The listing builds one solid part. Answer for the finished solid, in the listing's coordinates (mm). A direction names the side the tool comes from. Round coordinates to 2 decimals unless told otherwise and drop trailing zeros. Loops run counter-clockwise (first coordinate to the right, second up) from the corner with the lowest first, then second, coordinate; pieces in that order, holes last. Notation, with made-up numbers: (79, 32) -> (97, 32) arc R31 cw to (97, 56) -> close; hole circle Ø2 at (10, 24). An arc over 180 degrees is marked (long way). Write each question's results on one line, items separated by ' | '. Start each with the question number.
from build123d import *

# Parameters (mm, degrees)
F1_DEPTH = 40
F3_DEPTH = 260


with BuildPart() as f1:
    # F0 (on Top) → F1 (new body)
    with BuildSketch(Plane.XY):
        with BuildLine():
            Line((184.88144, 231.240067), (-175.11856, 231.240067))
            ThreePointArc((-175.11856, 231.240067), (-189.260696, 225.382203), (-195.11856, 211.240067))
            Line((-195.11856, 211.240067), (-195.11856, -148.759933))
            ThreePointArc((-195.11856, -148.759933), (-189.260696, -162.902068), (-175.11856, -168.759933))
            Line((-175.11856, -168.759933), (184.88144, -168.759933))
            ThreePointArc((184.88144, -168.759933), (199.023575, -162.902068), (204.88144, -148.759933))
            Line((204.88144, -148.759933), (204.88144, 211.240067))
            ThreePointArc((204.88144, 211.240067), (199.023575, 225.382203), (184.88144, 231.240067))
        make_face()
    extrude(amount=F1_DEPTH)

    # F2 (on face) → F3 (join)
    with BuildSketch(Plane(origin=(0, 0, 0), x_dir=(1, 0, 0), z_dir=(0, 0, -1))):
        with BuildLine():
            ThreePointArc((-135.11856, -191.240067), (-120.976425, -185.382203), (-115.11856, -171.240067))
            ThreePointArc((-115.11856, -171.240067), (-120.976425, -157.097932), (-135.11856, -151.240067))
            ThreePointArc((-135.11856, -151.240067), (-149.260696, -157.097932), (-155.11856, -171.240067))
            ThreePointArc((-155.11856, -171.240067), (-149.260696, -185.382203), (-135.11856, -191.240067))
        make_face()
        with BuildLine():
            ThreePointArc((-135.11856, 88.759933), (-120.976425, 94.617797), (-115.11856, 108.759933))
            ThreePointArc((-115.11856, 108.759933), (-120.976425, 122.902068), (-135.11856, 128.759933))
            ThreePointArc((-135.11856, 128.759933), (-149.260696, 122.902068), (-155.11856, 108.759933))
            ThreePointArc((-155.11856, 108.759933), (-149.260696, 94.617797), (-135.11856, 88.759933))
        make_face()
        with BuildLine():
            ThreePointArc((144.88144, 128.759933), (130.739304, 122.902068), (124.88144, 108.759933))
            ThreePointArc((124.88144, 108.759933), (130.739304, 94.617797), (144.88144, 88.759933))
            ThreePointArc((144.88144, 88.759933), (159.023575, 94.617797), (164.88144, 108.759933))
            ThreePointArc((164.88144, 108.759933), (159.023575, 122.902068), (144.88144, 128.759933))
        make_face()
        with BuildLine():
            ThreePointArc((164.88144, -171.240067), (159.023575, -157.097932), (144.88144, -151.240067))
            ThreePointArc((144.88144, -151.240067), (130.739304, -157.097932), (124.88144, -171.240067))
            ThreePointArc((124.88144, -171.240067), (130.739304, -185.382203), (144.88144, -191.240067))
            ThreePointArc((144.88144, -191.240067), (159.023575, -185.382203), (164.88144, -171.240067))
        make_face()
    extrude(amount=F3_DEPTH)


solid = f1.part
Item 1: The part is cut by section D-D, the plane x = 40.5. Give the vertices of the cut face in (y, z).
Item 2: The part is cut by section A-A, the plane z = -74. Give the vertices of the cut face in (x, y), plus the area to 3 significant figures.
Item 3: For faces 1 (the flat face through (2, 34, 0)), 2 (the flat face through (-135, -109, -260)), determine the directions among +Z, -Z, +X, -X, +Y, -Y from which every point of the face is accessible in a straight line to the end or side of a thin tool.
Item 4: The part is cut by section B-B, the plane y = 183.5. Give the vertices of the cut face in (x, z).
Item 5: Straight lines are drawn through the part: L1, parallel to X at y = 163.5, z = -160; L2, parallel to Z at x = 16, y = 91; L3, parallel to X at y = -96.5, z = -226.5. For each, find the intervals that lie inside material, in ascending order. Write a range as [from, to].
Item 6: The part is cut by section C-C, the plane x = 152. Give the vertices of the cut face in (y, z), plus the area to 3 significant figures.
Item 7: Each of these flat-tipped pins is pushed along its axis until it touches: pin 1 Ø12 at (x, z) = (145, -36.5) entering from +Y; pin 2 Ø4 at (x, y) = (24.5, 14) entering from -Z. Where does it stop, or does it pass through?
Report:
1) outline: (-168.76, 0) -> (231.24, 0) -> (231.24, 40) -> (-168.76, 40) -> close
2) outline: (-155.12, -108.76) arc R20 ccw to (-135.12, -128.76) arc R20 ccw to (-115.12, -108.76) arc R20 ccw to (-135.12, -88.76) arc R20 ccw to start; (-155.12, 171.24) arc R20 ccw to (-135.12, 151.24) arc R20 ccw to (-115.12, 171.24) arc R20 ccw to (-135.12, 191.24) arc R20 ccw to start; (124.88, -108.76) arc R20 ccw to (144.88, -128.76) arc R20 ccw to (164.88, -108.76) arc R20 ccw to (144.88, -88.76) arc R20 ccw to start; (124.88, 171.24) arc R20 ccw to (144.88, 151.24) arc R20 ccw to (164.88, 171.24) arc R20 ccw to (144.88, 191.24) arc R20 ccw to start | area: 5,030 mm2
3) face 1: -Z | face 2: -Z, +X, -X, +Y, -Y
4) outline: (-195.12, 0) -> (-150.92, 0) -> (-150.92, -260) -> (-119.32, -260) -> (-119.32, 0) -> (129.08, 0) -> (129.08, -260) -> (160.68, -260) -> (160.68, 0) -> (204.88, 0) -> (204.88, 40) -> (-195.12, 40) -> close
5) L1: x = [-153.56, -116.68], [126.44, 163.32] | L2: z = [0, 40] | L3: x = [-150.92, -119.32], [129.08, 160.68]
6) outline: (-168.76, 0) -> (-127.45, 0) -> (-127.45, -260) -> (-90.07, -260) -> (-90.07, 0) -> (152.55, 0) -> (152.55, -260) -> (189.93, -260) -> (189.93, 0) -> (231.24, 0) -> (231.24, 40) -> (-168.76, 40) -> close | area: 35,400 mm2
7) pin 1: stops at y = 191.24 | pin 2: stops at z = 0
